Part model, mm, in its own coordinate system. A direction names the side the tool comes from. Coordinates: 2 decimals unless noted, no trailing zeros. Order: outer loops, then holes, each group sorted by start corner. A loop starts at its lowest first (then second) coordinate and runs counter-clockwise, first axis right, second up. Notation, with made-up numbers: (88.5, -16) - (129.5, -16) arc R35 ccw to (129.5, 19) - close; hole circle Ø2 at (64.5, 11). An arc over 180 degrees is marked (long way). Use a Markdown table: item, result. Add a question column.
1) Tool access for faces 1 (the face through (45.78, 12.87, 1.48)), 2 (the face through (42, 18, 3)): list every direction of +Z, -Z, +X, -X, +Y, -Y with a clear straight run to the whole face (end or side of a thin tool).
2) Two-plate mould, pull along Y, no slides. Class faces 3 (the face through (77.5, 14, 1)), 4 (the face through (36.724, 12.331, 1.479)), 5 (the face through (49, 0, 1)): +Y half, -Y half, draft (parallel to the pull), parting line (faces both ways), or undercut.
3) Drop flat-ended pins along their axis: P1, Ø3.5, axis at x = 63.5, y = 14.37, coming from the +Z side; P2, Ø3.5, axis at x = 22.5, y = 14.37, coming from the +Z side. Give the stop position or say it passes through.
4) Saw through at A-A on x = 20.5. List the corners of the cut face in (y, z).
5) Saw through at B-B on y = 22.5. List the corners of the cut face in (x, z), then the cut area to 3 significant figures.
6) Wall check: L1, parallel to X at y = 17.5, z = 1; L2, parallel to X at y = 10.25, z = 1.95; L3, parallel to X at y = 16, z = 0.85. Give the ranges that are in metal, low to high. Write a range as [from, to].
7) Saw through at D-D on y = 8.75. List the corners of the cut face in (x, z), then the cut area to 3 significant figures.
8) Saw through at C-C on x = 54. List the corners of the cut face in (y, z).
```python
from build123d import *

# Parameters (mm, degrees)
F0_R     = 3
F0_R_2   = 1.6
F1_DEPTH = 3
F2_R     = 1


with BuildPart() as f1:
    # F0 (on Top) → F1 (new body)
    with BuildSketch(Plane.XY):
        with BuildLine():
            ThreePointArc((22.499999, 28.739418), (8.13029, 14.36971), (22.499997, 0))
            Line((22.499997, 0), (77.499997, 0))
            Line((77.499997, 0), (77.499999, 28.739418))
            Line((77.499999, 28.739418), (22.499999, 28.739418))
        make_face()
        with Locations((22.499999, 14.369709)):
            Circle(F0_R, mode=Mode.SUBTRACT)
        with BuildLine():
            Line((35.480354, 20.534036), (56.380585, 4.982745))
            Line((56.380585, 4.982745), (33.379955, 4.982745))
            ThreePointArc((33.379955, 4.982745), (36.740409, 12.446362), (35.480354, 20.534036))
        make_face(mode=Mode.SUBTRACT)
        with Locations((63.499998, 14.369709)):
            Circle(F0_R_2, mode=Mode.SUBTRACT)
        with Locations((71.499998, 14.369709)):
            Circle(F0_R_2, mode=Mode.SUBTRACT)
        Polygon((36.174804, 23.756673), (58.893349, 23.756673), (58.893349, 6.852424), align=None, mode=Mode.SUBTRACT)
    extrude(amount=F1_DEPTH)

    # F2
    f2_edges = [f1.edges().sort_by_distance(p)[0] for p in [
        (77.499997, 0, 1.5),
        (77.499999, 28.739418, 1.5),
    ]]
    fillet(f2_edges, radius=F2_R)


solid = f1.part
```
Results are:
| question | item | result |
|---|---|---|
| 1 | face 1 | +Z, -Z |
| 1 | face 2 | +Z, +X, -X, +Y, -Y |
| 2 | face 3 | draft |
| 2 | face 4 | undercut |
| 2 | face 5 | -Y half |
| 3 | P1 | z = 3 |
| 3 | P2 | through |
| 4 | outline | (0.14, 0) - (12.13, 0) - (12.13, 3) - (0.14, 3) - close; (16.61, 0) - (28.6, 0) - (28.6, 3) - (16.61, 3) - close |
| 5 | outline | (10.65, 0) - (37.86, 0) - (37.86, 3) - (10.65, 3) - close; (58.89, 0) - (77.5, 0) - (77.5, 3) - (58.89, 3) - close |
| 5 | area | 137 mm2 |
| 6 | L1 | [8.48, 36.52], [39.56, 44.58], [58.89, 77.5] |
| 6 | L2 | [8.73, 36.27], [49.3, 54.33], [58.89, 77.5] |
| 6 | L3 | [8.22, 19.98], [25.02, 36.78], [41.57, 46.6], [58.89, 77.5] |
| 7 | outline | (9.27, 0) - (35.73, 0) - (35.73, 3) - (9.27, 3) - close; (51.32, 0) - (56.34, 0) - (56.34, 3) - (51.32, 3) - close; (58.89, 0) - (77.5, 0) - (77.5, 3) - (58.89, 3) - close |
| 7 | area | 150 mm2 |
| 8 | outline | (0, 0) - (4.98, 0) - (4.98, 3) - (0, 3) - close; (6.75, 0) - (10.49, 0) - (10.49, 3) - (6.75, 3) - close; (23.76, 0) - (28.74, 0) - (28.74, 3) - (23.76, 3) - close |
